from build123d import *

# Parameters (mm, degrees)
F0_W          = 70
F0_H          = 90
F1_DEPTH      = 3
F2_D          = 52
F3_R          = 26
F3_R_2        = 12.5
F4_DEPTH      = 9
F4_DEPTH_BACK = 6
F5_W          = 40
F5_H          = 15
F6_DEPTH      = 25


with BuildPart() as f1:
    # F0 (on Front) → F1 (new body)
    with BuildSketch(Plane.XZ):
        Rectangle(F0_W, F0_H)
    extrude(amount=F1_DEPTH)

    # F2 (through all)
    with Locations(Plane(origin=(0, 0, 0), x_dir=(1, 0, 0), z_dir=(0, 1, 0))):
        with Locations((0, 0)):
            Hole(F2_D / 2)

    # F3 (on Front) → F4 (join, two sides)
    with BuildSketch(Plane.XZ) as f4_sk:
        Circle(F3_R)
        Circle(F3_R_2, mode=Mode.SUBTRACT)
    extrude(amount=F4_DEPTH)
    extrude(f4_sk.sketch, amount=-F4_DEPTH_BACK)

    # F5 (on face) → F6 (cut)
    with BuildSketch(Plane.XZ.offset(3)):
        with Locations((0, 37.5)):
            Rectangle(F5_W, F5_H)
    extrude(amount=-F6_DEPTH, mode=Mode.SUBTRACT)


solid = f1.part
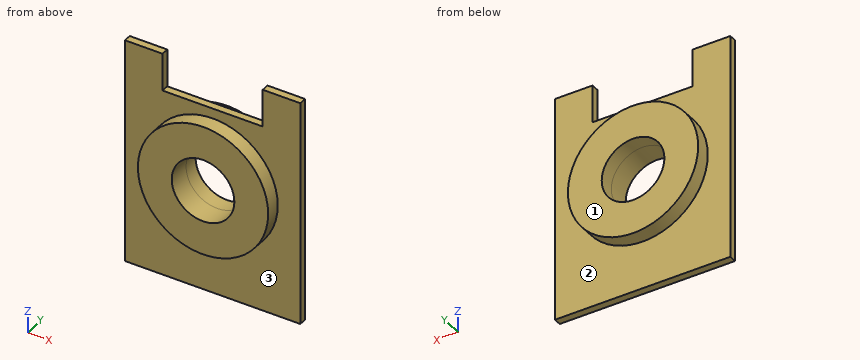
For this review, take the finished solid that the model builds, in its own axes (mm). Face numbers are marked on the shaded views. A direction names the side the tool comes from. Give positions to 0.01 mm unless a question says otherwise; leave off trailing zeros. Write each loop counter-clockwise with the first axis right and the second up, starting at its lowest first coordinate (ties: lowest second). Pieces come first, ordered by that corner, then holes. Notation, with made-up numbers: (59.25, 5) -> (110.25, 5) arc R14 cw to (110.25, 31) -> close; hole circle Ø4 at (-16, 53.5). An arc over 180 degrees is marked (long way). Use CSV: the item, a comma, the result in double quotes.
Q1. Take a section at C-C, the plane y = -4.5. Write out the cut boundary in (x, z), then the cut area to 3 significant figures.
Conclusion:
outline,"circle Ø52 at (0, 0); hole circle Ø25 at (0, 0)"
area,"1,630 mm2"
Q2. To check wall thickness, follow probe 1 along Z at (x, y) = (0, -3.5); probe 2 along Z at (x, y) = (0, -2); probe 3 along X at (y, z) = (-1.5, 41). State the ranges of each line that lie inside material, in increasing order. Write a range as [from, to].
Conclusion:
probe 1,"[-26, -12.5], [12.5, 26]"
probe 2,"[-45, -12.5], [12.5, 30]"
probe 3,"[-35, -20], [20, 35]"
Q3. For P1, Ø8, axis at x = 2, y = -5.5, coming from the +Z side; P2, Ø1.5, axis at x = 14, y = 4.5, coming from the -Z side; P3, Ø1.5, axis at y = 3, z = 21, coming from the -X side, all flat-tipped, find the tip position at first contact; note any pin that passes through.
Conclusion:
P1,"z = 30"
P2,"z = -22.37"
P3,"x = -16.31"
Q4. Take a section at D-D, the plane x = -21. Write out the cut boundary in (y, z), then the cut area to 3 significant figures.
Conclusion:
outline,"(-9, -15.33) -> (-3, -15.33) -> (-3, -45) -> (0, -45) -> (0, -15.33) -> (6, -15.33) -> (6, 15.33) -> (0, 15.33) -> (0, 45) -> (-3, 45) -> (-3, 15.33) -> (-9, 15.33) -> close"
area,"638 mm2"
Q5. Tool access review of the marked faces 1, 2 and 3: name each direction out of +Z, -Z, +X, -X, +Y, -Y from which nothing blocks a thin tool from reaching the whole face with its end or side.
Conclusion:
face 1,"+Z, -Z, +X, -X, +Y"
face 2,"+Y"
face 3,"-Y"
Q6. Take a section at A-A, the plane z = 0. Write out the cut boundary in (x, y), then the cut area to 3 significant figures.
Conclusion:
outline,"(-35, -3) -> (-26, -3) -> (-26, -9) -> (-12.5, -9) -> (-12.5, 6) -> (-26, 6) -> (-26, 0) -> (-35, 0) -> close; (12.5, -9) -> (26, -9) -> (26, -3) -> (35, -3) -> (35, 0) -> (26, 0) -> (26, 6) -> (12.5, 6) -> close"
area,"459 mm2"
Q7. Take a section at B-B, the plane x = 0. Write out the cut boundary in (y, z), then the cut area to 3 significant figures.
Conclusion:
outline,"(-9, -26) -> (-3, -26) -> (-3, -45) -> (0, -45) -> (0, -26) -> (6, -26) -> (6, -12.5) -> (-9, -12.5) -> close; (-9, 12.5) -> (6, 12.5) -> (6, 26) -> (0, 26) -> (0, 30) -> (-3, 30) -> (-3, 26) -> (-9, 26) -> close"
area,"474 mm2"
